The model under review builds one solid part; all positions refer to its coordinate system, in mm. A direction names the side the tool comes from. Coordinates: 2 decimals unless noted, no trailing zeros. Order: outer loops, then holes, each group sorted by start corner. A loop starts at its lowest first (then second) coordinate and runs counter-clockwise, first axis right, second up. Notation, with made-up numbers: M 17.5,58.25 L 31.5,58.25 A32 ccw 31.5,95.25 Z; hole C 30,53 d1. An arc over 180 degrees is marked long. One line per item, written item: value.
Autodesk Inventor part; units mm, degrees
ref_plane "YZ Plane" through (0, 0, 0) normal (1, 0, 0) x (0, 1, 0)
ref_plane "XZ Plane" through (0, 0, 0) normal (0, 1, 0) x (-1, 0, 0)
ref_plane "XY Plane" through (0, 0, 0) normal (0, 0, 1) x (1, 0, 0)
sketch "Эскиз1" plane through (0, 0, 0) normal (0, 1, 0) x (-1, 0, 0)
  line L0 (0, 0) -> (15, 0)
  line L1 (15, 0) -> (15, -30)
  line L2 (15, -30) -> (0, -30)
  line L3 (0, -30) -> (0, 0)
  line L4 (13, -2) -> (8.5, -2)
  line L5 (8.5, -2) -> (8.5, -6.5)
  line L6 (8.5, -6.5) -> (13, -6.5)
  line L7 (13, -6.5) -> (13, -2)
  line L8 (13, -7.375) -> (8.5, -7.375)
  line L9 (8.5, -7.375) -> (8.5, -11.875)
  line L10 (8.5, -11.875) -> (13, -11.875)
  line L11 (13, -11.875) -> (13, -7.375)
  line L12 (13, -12.75) -> (8.5, -12.75)
  line L13 (8.5, -12.75) -> (8.5, -17.25)
  line L14 (8.5, -17.25) -> (13, -17.25)
  line L15 (13, -17.25) -> (13, -12.75)
  line L16 (13, -18.125) -> (8.5, -18.125)
  line L17 (8.5, -18.125) -> (8.5, -28)
  line L18 (8.5, -28) -> (13, -28)
  line L19 (13, -28) -> (13, -18.125)
  line L20 (6.5, -18.125) -> (2, -18.125)
  line L21 (2, -18.125) -> (2, -22.625)
  line L22 (2, -22.625) -> (6.5, -22.625)
  line L23 (6.5, -22.625) -> (6.5, -18.125)
  line L24 (6.5, -23.5) -> (2, -23.5)
  line L25 (2, -23.5) -> (2, -28)
  line L26 (2, -28) -> (6.5, -28)
  line L27 (6.5, -28) -> (6.5, -23.5)
  line L28 (6.5, -2) -> (2, -2)
  line L29 (2, -2) -> (2, -17.25)
  line L30 (2, -17.25) -> (6.5, -17.25)
  line L31 (6.5, -17.25) -> (6.5, -2)
  line L32 (10.75, -6.5) -> (10.75, -7.375)
  line L33 (10.75, -11.875) -> (10.75, -12.75)
  line L34 (10.75, -17.25) -> (10.75, -18.125)
  line L35 (4.25, -17.25) -> (4.25, -18.125)
  line L36 (4.25, -22.625) -> (4.25, -23.5)
  line L37 (10.75, -2) -> (10.75, 0)
  line L38 (10.75, -28) -> (10.75, -30)
  line L39 (13, -9.625) -> (15, -9.625)
  line L40 (2, -9.625) -> (0, -9.625)
  line L41 (8.5, -9.625) -> (6.5, -9.625)
  dimension "d0" = 15
  dimension "d1" = 30
  dimension "d9" = 2
extrude "Выдавливание1" add sketch "Эскиз1" along normal blind 1 contours L0 L37 L4 L5 L6 L32 L8 L9 L41 L31 L28 L29 L40 L3 | L0 L1 L39 L11 L8 L32 L6 L7 L4 L37 | L40 L29 L30 L31 L41 L9 L10 L33 L12 L13 L14 L34 L16 L17 L18 L38 L2 L3 | L1 L2 L38 L18 L19 L16 L34 L14 L15 L12 L33 L10 L11 L39
sketch "Эскиз2" plane through (0, 0, 0) normal (0, -1, 0) x (1, 0, 0)
  line L0 (0, 0) -> (0, -30)
  line L1 (-15, 0) -> (0, 0)
  line L2 (-15, -30) -> (-15, 0)
  line L3 (0, -30) -> (-15, -30)
  line L4 (-6.5, -17.25) -> (-2, -17.25)
  line L5 (-6.5, -2) -> (-6.5, -17.25)
  line L6 (-2, -2) -> (-6.5, -2)
  line L7 (-2, -17.25) -> (-2, -2)
  line L8 (-2, -28) -> (-2, -23.5)
  line L9 (-6.5, -28) -> (-2, -28)
  line L10 (-6.5, -23.5) -> (-6.5, -28)
  line L11 (-2, -23.5) -> (-6.5, -23.5)
  line L12 (-8.5, -12.75) -> (-13, -12.75)
  line L13 (-8.5, -17.25) -> (-8.5, -12.75)
  line L14 (-13, -17.25) -> (-8.5, -17.25)
  line L15 (-13, -12.75) -> (-13, -17.25)
  line L16 (-13, -18.125) -> (-13, -28)
  line L17 (-8.5, -18.125) -> (-13, -18.125)
  line L18 (-8.5, -28) -> (-8.5, -18.125)
  line L19 (-13, -28) -> (-8.5, -28)
  line L20 (-13, -11.875) -> (-8.5, -11.875)
  line L21 (-13, -7.375) -> (-13, -11.875)
  line L22 (-8.5, -7.375) -> (-13, -7.375)
  line L23 (-8.5, -11.875) -> (-8.5, -7.375)
  line L24 (-13, -2) -> (-13, -6.5)
  line L25 (-8.5, -2) -> (-13, -2)
  line L26 (-8.5, -6.5) -> (-8.5, -2)
  line L27 (-13, -6.5) -> (-8.5, -6.5)
  line L28 (-2, -22.625) -> (-2, -18.125)
  line L29 (-6.5, -22.625) -> (-2, -22.625)
  line L30 (-6.5, -18.125) -> (-6.5, -22.625)
  line L31 (-2, -18.125) -> (-6.5, -18.125)
extrude "Выдавливание2" add sketch "Эскиз2" along normal blind 1 contours L0 L3 L2 L1 | L5 L6 L7 L4 | L9 L10 L11 L8 | L13 L14 L15 L12 | L17 L18 L19 L16 | L21 L22 L23 L20 | L25 L26 L27 L24 | L29 L30 L31 L28
sketch "Эскиз3" plane through (-15, 1, 0) normal (0, 0, 1) x (1, 0, 0)
  line L0 (0, -2) -> (15, -2)
  line L1 (15, -2) -> (15, -1)
  line L2 (15, -1) -> (0, -1)
  line L3 (0, -1) -> (0, -2)
  line L4 (15, -2) -> (15, 0)
  line L5 (0, -2) -> (0, 0)
  line L6 (15, -2) -> (0, -2)
  dimension "d14" = 1
extrude "Выдавливание3" add sketch "Эскиз3" along normal blind 1
sketch "Эскиз4" plane through (0, 1, -30) normal (0, 0, -1) x (-1, 0, 0)
  line L0 (8.5, -1) -> (13, -1)
  line L1 (15, -2) -> (0, -2)
  line L2 (0, -2) -> (0, -1)
  line L3 (0, -1) -> (15, -1)
  line L4 (15, -1) -> (15, -2)
extrude "Выдавливание4" add sketch "Эскиз4" along normal blind 1
properties part number "Лого ШП"
(1) We need section A-A, the plane z = -21. State the section outline as (x, y) points.
Geometry results:
outline: M -15,-1 L 0,-1 L 0,1 L -2,1 L -2,0 L -6.5,0 L -6.5,1 L -8.5,1 L -8.5,0 L -13,0 L -13,1 L -15,1 Z
(2) Tool access review of faces 4 (the flat face through (-7, 1, -15)), 5 (the flat face through (-13, 0.5, -15)), 6 (the flat face through (-7.4, 0, 0.5)): name each direction out of +Z, -Z, +X, -X, +Y, -Y from which nothing blocks a thin tool from reaching the whole face with its end or side.
Geometry results:
face 4: +Z, -Z, +X, -X, +Y
face 5: +Y
face 6: +Z, +X, -X, +Y
(3) We need section B-B, the plane y = 0.6. Count the separate pieces of the cut face and the enclosed holes in it, plus the area to 3 significant figures.
Geometry results:
separate pieces: 1
enclosed holes: 7
area: 236 mm2
(4) We need section D-D, the plane x = -3.25. State the section outline as (y, z) points (3 decimals).
Geometry results:
outline: M -1,-31 L 0,-31 L 0,-30 L 1,-30 L 1,-28 L 0,-28 L 0,-23.5 L 1,-23.5 L 1,-22.625 L 0,-22.625 L 0,-18.125 L 1,-18.125 L 1,-17.25 L 0,-17.25 L 0,-2 L 1,-2 L 1,0 L 0,0 L 0,1 L -1,1 Z
(5) Insertion check: pin 1 Ø0.5 at (x, y) = (-7.5, 0.5) entering from -Z; pin 2 Ø1.3 at (x, z) = (-10.5, -9) entering from +Y; pin 3 Ø0.5 at (x, y) = (-12, 0.5) entering from +Z. Each pin has a flat end and moves straight along its axis. Give the tip position at first contact, or say it passes through.
Geometry results:
pin 1: stops at z = -30
pin 2: stops at y = 0
pin 3: stops at z = 0
(6) We need section C-C, the plane x = -9. State the section outline as (y, z) points (3 decimals).
Geometry results:
outline: M -1,-31 L 0,-31 L 0,-30 L 1,-30 L 1,-28 L 0,-28 L 0,-18.125 L 1,-18.125 L 1,-17.25 L 0,-17.25 L 0,-12.75 L 1,-12.75 L 1,-11.875 L 0,-11.875 L 0,-7.375 L 1,-7.375 L 1,-6.5 L 0,-6.5 L 0,-2 L 1,-2 L 1,0 L 0,0 L 0,1 L -1,1 Z
(7) For L1, parallel to Z at x = -5.75, y = 0.35 (3 decimals); L2, parallel to X at y = 0.25, z = -27; L3, parallel to Y at x = -9.75, z = -11, list the stretches that pass through material, from the lowest coordinate up.
Geometry results:
L1: z = -30 to -28, -23.5 to -22.625, -18.125 to -17.25, -2 to 0
L2: x = -15 to -13, -8.5 to -6.5, -2 to 0
L3: y = -1 to 0
(8) Mouldability with a two-part tool opening along X and no side actions: class faces 1 (the flat face through (0, 0, -15)), 2 (the flat face through (-8, -1, -15)), 3 (the flat face through (-10.7, 0.5, -17.25)) as +X half, -X half, draft (parallel to the pull), parting line (faces both ways), or undercut.
Geometry results:
face 1: +X half
face 2: draft
face 3: undercut
